from build123d import *

# Parameters (mm, degrees)
F0_W     = 38.1
F0_H     = 31.75
F1_DEPTH = 6.35
F3_D     = 2.5
F5_DEPTH = 12.7


# Not quite as in the source:
# - a pattern or mirror of a feature is missing from the dataset's text; its kind, count and spacing are read off the source's solid


with BuildPart() as f1:
    # F0 (on Front) → F1 (new body, symmetric)
    with BuildSketch(Plane.XZ):
        Rectangle(F0_W, F0_H)
    extrude(amount=F1_DEPTH, both=True)

    # F3 (through all)
    with Locations(Plane.XZ.offset(6.35)):
        with Locations((-10.99693, 2.7813), (11.10107, 13.081), (-10.99693, 13.081), (11.10107, 2.7813)):
            Hole(F3_D / 2)

    # F4 (on face) → F5 (cut, through all)
    with BuildSketch(Plane.XZ.offset(6.35)):
        with BuildLine():
            ThreePointArc((-10.45, -5.715), (-12.7, -3.465), (-14.95, -5.715))
            Line((-14.95, -5.715), (-14.95, -10.795))
            ThreePointArc((-14.95, -10.795), (-12.7, -13.045), (-10.45, -10.795))
            Line((-10.45, -10.795), (-10.45, -5.715))
        make_face()
    f5 = extrude(amount=-F5_DEPTH, mode=Mode.SUBTRACT)

    # F5_copies: F5 across plane
    add(f5.mirror(Plane(origin=(0, 0, 0), x_dir=(0, 0, 1), z_dir=(1, 0, 0))), mode=Mode.SUBTRACT)


solid = f1.part
Here's how the part is built. I have some questions about the finished solid (model axes, mm). A direction names the side the tool comes from. Coordinates: 2 decimals unless noted, no trailing zeros. Order: outer loops, then holes, each group sorted by start corner. A loop starts at its lowest first (then second) coordinate and runs counter-clockwise, first axis right, second up. Notation, with made-up numbers: (13.25, 44) -> (25.25, 44) arc R19 ccw to (25.25, 64) -> close; hole circle Ø5 at (32, 52.25). An arc over 180 degrees is marked (long way). Answer in a Markdown table with one row per item.
(1) Thinking about a two-plate mould opening in X: for faces 1 (the face through (12.749, -0.089, -13.044)), 2 (the face through (19.05, 0, 0)), 3 (the face through (0, 6.35, 0)), which applies, +X half, -X half, draft (parallel to the pull), parting line (faces both ways), or undercut?
Answer key:
| item | result |
|---|---|
| face 1 | undercut |
| face 2 | +X half |
| face 3 | draft |
(2) I want a section at B-B on y = 5. List the corners of the cut face in (x, z) for me (3 decimals), then the cut area to 3 significant figures.
Answer key:
| item | result |
|---|---|
| outline | (-19.05, -15.875) -> (19.05, -15.875) -> (19.05, 15.875) -> (-19.05, 15.875) -> close; hole (-14.95, -10.795) arc R2.25 ccw to (-10.45, -10.795) -> (-10.45, -5.715) arc R2.25 ccw to (-14.95, -5.715) -> close; hole circle Ø2.5 at (-10.997, 2.781); hole circle Ø2.5 at (-10.997, 13.081); hole circle Ø2.5 at (11.101, 2.781); hole circle Ø2.5 at (11.101, 13.081); hole (10.45, -10.795) arc R2.25 ccw to (14.95, -10.795) -> (14.95, -5.715) arc R2.25 ccw to (10.45, -5.715) -> close |
| area | 1,110 mm^2 |
(3) Please list where these lines run through material, in increasing order: probe 1 along X at (y, z) = (5.75, -7); probe 2 along X at (y, z) = (2.5, 14); probe 3 along Z at (x, y) = (-13.5, 1.5) (3 decimals).
Answer key:
| item | result |
|---|---|
| probe 1 | -19.05 to -14.95, -10.45 to 10.45, 14.95 to 19.05 |
| probe 2 | -19.05 to -11.84, -10.15 to 10.25, 11.95 to 19.05 |
| probe 3 | -15.875 to -12.898, -3.612 to 15.875 |
(4) Will this pin go through, and if not, where does the flat tip stop? pin 1 Ø1.5 at (x, z) = (11.1, 2.78) entering from -Y.
Answer key:
| item | result |
|---|---|
| pin 1 | through |
(5) I want a section at A-A on x = -12.7. List the corners of the cut face in (y, z) for me (3 decimals).
Answer key:
| item | result |
|---|---|
| outline | (-6.35, -15.875) -> (6.35, -15.875) -> (6.35, -13.045) -> (-6.35, -13.045) -> close; (-6.35, -3.465) -> (6.35, -3.465) -> (6.35, 15.875) -> (-6.35, 15.875) -> close |
(6) On a 3-axis mill with a long thin cutter (end or side, diameter ignored), from which of +Z, -Z, +X, -X, +Y, -Y can I reach the whole of each face in a straight line? I mean faces 4 (the face through (-19.05, 0, 0)), 5 (the face through (-12.651, -0.089, -3.466)). Say none if no direction works.
Answer key:
| item | result |
|---|---|
| face 4 | +Z, -Z, -X, +Y, -Y |
| face 5 | +Y, -Y |
